The listing builds one solid part. Answer for the finished solid, in the listing's coordinates (mm). Face numbers are marked on the shaded views. Coordinates: 2 decimals unless noted, no trailing zeros. Write each loop counter-clockwise with the first axis right and the second up, starting at its lowest first coordinate (ties: lowest second). Pieces come first, ordered by that corner, then holes.
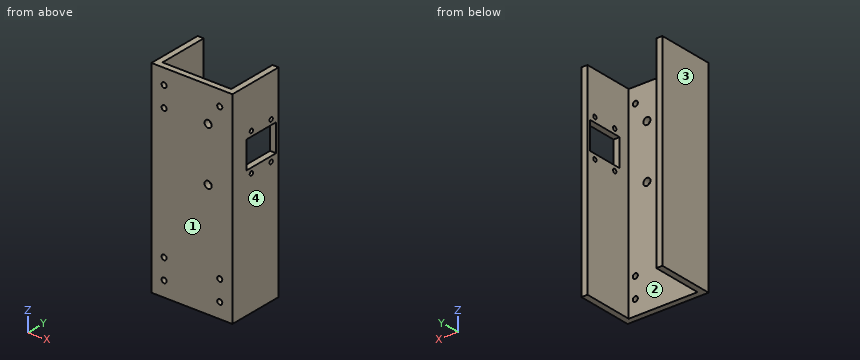
```python
from build123d import *

# Parameters (mm, degrees)
EXTRUDE_1_DEPTH     = 200
CUT_EXTRUDE_2_REACH = 58
SKETCH_4_R          = 2.5
SKETCH_8_R          = 2
SKETCH_8_W          = 27
SKETCH_8_H          = 36
CUT_EXTRUDE_5_DEPTH = 10
SKETCH_9_R          = 3.5
CUT_EXTRUDE_6_DEPTH = 10
SKETCH_10_R         = 3.500000002
SKETCH_10_R_2       = 3.5
CUT_EXTRUDE_7_DEPTH = 10


with BuildPart() as part:
    # 草图1 → 凸台-拉伸1 (new body)
    with BuildSketch(Plane.XY):
        Polygon((-40, 0), (40, 0), (40, 56), (34, 56), (34, 6), (-34, 6), (-34, 56), (-40, 56), align=None)
    extrude(amount=EXTRUDE_1_DEPTH)

    # 草图4 → 切除-拉伸2 (cut, up to next)
    with BuildSketch(Plane.XZ, mode=Mode.PRIVATE) as cut_extrude_2_sk1:
        with Locations((-27.5, 185)):
            Circle(SKETCH_4_R)
    cut_extrude_2_tool1 = extrude(cut_extrude_2_sk1.sketch, amount=-CUT_EXTRUDE_2_REACH, mode=Mode.PRIVATE) & part.part
    add(cut_extrude_2_tool1.solids().sort_by_distance((-27.5, 0, 185))[0], mode=Mode.SUBTRACT)
    # 草图4 → 切除-拉伸2 (cut, up to next)
    with BuildSketch(Plane.XZ, mode=Mode.PRIVATE) as cut_extrude_2_sk2:
        with Locations((27.5, 185)):
            Circle(SKETCH_4_R)
    cut_extrude_2_tool2 = extrude(cut_extrude_2_sk2.sketch, amount=-CUT_EXTRUDE_2_REACH, mode=Mode.PRIVATE) & part.part
    add(cut_extrude_2_tool2.solids().sort_by_distance((27.5, 0, 185))[0], mode=Mode.SUBTRACT)
    # 草图4 → 切除-拉伸2 (cut, up to next)
    with BuildSketch(Plane.XZ, mode=Mode.PRIVATE) as cut_extrude_2_sk3:
        with Locations((-27.5, 165)):
            Circle(SKETCH_4_R)
    cut_extrude_2_tool3 = extrude(cut_extrude_2_sk3.sketch, amount=-CUT_EXTRUDE_2_REACH, mode=Mode.PRIVATE) & part.part
    add(cut_extrude_2_tool3.solids().sort_by_distance((-27.5, 0, 165))[0], mode=Mode.SUBTRACT)
    # 草图4 → 切除-拉伸2 (cut, up to next)
    with BuildSketch(Plane.XZ, mode=Mode.PRIVATE) as cut_extrude_2_sk4:
        with Locations((27.5, 35)):
            Circle(SKETCH_4_R)
    cut_extrude_2_tool4 = extrude(cut_extrude_2_sk4.sketch, amount=-CUT_EXTRUDE_2_REACH, mode=Mode.PRIVATE) & part.part
    add(cut_extrude_2_tool4.solids().sort_by_distance((27.5, 0, 35))[0], mode=Mode.SUBTRACT)
    # 草图4 → 切除-拉伸2 (cut, up to next)
    with BuildSketch(Plane.XZ, mode=Mode.PRIVATE) as cut_extrude_2_sk5:
        with Locations((-27.5, 35)):
            Circle(SKETCH_4_R)
    cut_extrude_2_tool5 = extrude(cut_extrude_2_sk5.sketch, amount=-CUT_EXTRUDE_2_REACH, mode=Mode.PRIVATE) & part.part
    add(cut_extrude_2_tool5.solids().sort_by_distance((-27.5, 0, 35))[0], mode=Mode.SUBTRACT)
    # 草图4 → 切除-拉伸2 (cut, up to next)
    with BuildSketch(Plane.XZ, mode=Mode.PRIVATE) as cut_extrude_2_sk6:
        with Locations((27.5, 15)):
            Circle(SKETCH_4_R)
    cut_extrude_2_tool6 = extrude(cut_extrude_2_sk6.sketch, amount=-CUT_EXTRUDE_2_REACH, mode=Mode.PRIVATE) & part.part
    add(cut_extrude_2_tool6.solids().sort_by_distance((27.5, 0, 15))[0], mode=Mode.SUBTRACT)
    # 草图4 → 切除-拉伸2 (cut, up to next)
    with BuildSketch(Plane.XZ, mode=Mode.PRIVATE) as cut_extrude_2_sk7:
        with Locations((-27.5, 15)):
            Circle(SKETCH_4_R)
    cut_extrude_2_tool7 = extrude(cut_extrude_2_sk7.sketch, amount=-CUT_EXTRUDE_2_REACH, mode=Mode.PRIVATE) & part.part
    add(cut_extrude_2_tool7.solids().sort_by_distance((-27.5, 0, 15))[0], mode=Mode.SUBTRACT)

    # 草图8 → 切除-拉伸5 (cut)
    with BuildSketch(Plane(origin=(40, 0, 0), x_dir=(0, 0, -1), z_dir=(1, 0, 0))):
        with Locations((-121.5, 23)):
            Circle(SKETCH_8_R)
        with Locations((-121.5, 47)):
            Circle(SKETCH_8_R)
        with Locations((-158.5, 47)):
            Circle(SKETCH_8_R)
        with Locations((-158.5, 23)):
            Circle(SKETCH_8_R)
        with Locations((-140, 35)):
            Rectangle(SKETCH_8_W, SKETCH_8_H)
    extrude(amount=-CUT_EXTRUDE_5_DEPTH, mode=Mode.SUBTRACT)

    # 草图9 → 切除-拉伸6 (cut)
    with BuildSketch(Plane(origin=(0, 6, 0), x_dir=(1, 0, 0), z_dir=(0, 1, 0))):
        with Locations((15.999999998, -166)):
            Circle(SKETCH_9_R)
    extrude(amount=-CUT_EXTRUDE_6_DEPTH, mode=Mode.SUBTRACT)

    # 草图10 → 切除-拉伸7 (cut)
    with BuildSketch(Plane(origin=(0, 6, 0), x_dir=(1, 0, 0), z_dir=(0, 1, 0))):
        with Locations((15.999999998, -113)):
            Circle(SKETCH_10_R)
        with Locations((15.999999998, -166)):
            Circle(SKETCH_10_R_2)
    extrude(amount=-CUT_EXTRUDE_7_DEPTH, mode=Mode.SUBTRACT)


solid = part.part
```
(1) Section D-D, the plane x = 27.5 is taken. Write down the section's boundary in (y, z), plus the area to 3 significant figures.
(2) Section C-C, the plane x = -27.5 is taken. Write down the section's boundary in (y, z).
(3) Find the intervals of material crossed by probe 1 along Z at (x, y) = (-27.5, 3.7); probe 2 along X at (y, z) = (41, 124); probe 3 along X at (y, z) = (3.5, 113), in increasing order.
(4) For a pull along X with two mould halves and no side action, classify the marked faces 1, 2, 3 and 4 as pulls with the +X half, pulls with the -X half, needs draft (parallel to the pull), parting line crosses it, or undercut.
(5) Each of these flat-tipped pins is pushed along its axis until it touches: pin 1 (4 mm diameter, centred on x = -27.5, z = 15, fed in from -Y); pin 2 (8 mm diameter, centred on x = 27.5, z = 15, fed in from +Y); pin 3 (5 mm diameter, centred on x = 38, z = 141, fed in from -Y). Where does it stop, or does it pass through?
(6) Section A-A, the plane z = 121.5 is taken. Write down the section's boundary in (x, y).
(7) Section B-B, the plane y = 37 is taken. Write down the section's boundary in (x, z), plus the area to 3 significant figures.
Solution:
1. outline: (0, 0) - (6, 0) - (6, 12.5) - (0, 12.5) - close; (0, 17.5) - (6, 17.5) - (6, 32.5) - (0, 32.5) - close; (0, 37.5) - (6, 37.5) - (6, 182.5) - (0, 182.5) - close; (0, 187.5) - (6, 187.5) - (6, 200) - (0, 200) - close
1. area: 1,110 mm2
2. outline: (0, 0) - (6, 0) - (6, 12.5) - (0, 12.5) - close; (0, 17.5) - (6, 17.5) - (6, 32.5) - (0, 32.5) - close; (0, 37.5) - (6, 37.5) - (6, 162.5) - (0, 162.5) - close; (0, 167.5) - (6, 167.5) - (6, 182.5) - (0, 182.5) - close; (0, 187.5) - (6, 187.5) - (6, 200) - (0, 200) - close
3. probe 1: z = 0 to 12.5, 17.5 to 32.5, 37.5 to 162.5, 167.5 to 182.5, 187.5 to 200
3. probe 2: x = -40 to -34, 34 to 40
3. probe 3: x = -40 to 12.5, 19.5 to 40
4. face 1: needs draft
4. face 2: undercut
4. face 3: pulls with the -X half
4. face 4: pulls with the +X half
5. pin 1: passes through
5. pin 2: stops at y = 6
5. pin 3: stops at y = 0
6. outline: (-40, 0) - (40, 0) - (40, 21) - (34, 21) - (34, 6) - (-34, 6) - (-34, 56) - (-40, 56) - close; (34, 25) - (40, 25) - (40, 45) - (34, 45) - close; (34, 49) - (40, 49) - (40, 56) - (34, 56) - close
7. outline: (-40, 0) - (-34, 0) - (-34, 200) - (-40, 200) - close; (34, 0) - (40, 0) - (40, 126.5) - (34, 126.5) - close; (34, 153.5) - (40, 153.5) - (40, 200) - (34, 200) - close
7. area: 2,240 mm2
